Job drawing, mm, ordinate dimensions from the low corner. One solid piece. Give positions to 0.01 mm unless a question says otherwise; leave off trailing zeros. Order: outer loops, then holes, each group sorted by start corner. A loop starts at its lowest first (then second) coordinate and runs counter-clockwise, first axis right, second up. Notation, with made-up numbers: M 77,-21 L 119,-21 A17 cw 119,-8 Z; hole C 77.25,2 d2. An arc over 180 degrees is marked long. Put each result on its own line as item: value. Start each with the question number.
1) Cut at C-C (y = 16). Write the cut outline in (x, z) (1 decimal).
2) Cut at A-A (x = 17.5). Write the cut outline in (y, z).
3) Two-plate mould, pull along X, no slides. Class the marked faces 1, 2 and 3: released by +X, released by -X, zero draft, split by the parting line, or undercut.
4) Pin check, flat tips, straight feed: pin 1 (1.5 mm diameter, centred on x = 5.5, z = 22.5, fed in from -Y); pin 2 (12 mm diameter, centred on x = 21.5, z = 53, fed in from -Y); pin 3 (12 mm diameter, centred on x = 6.5, z = 60.5, fed in from -Y); pin 4 (10 mm diameter, centred on y = 54.5, z = 7, fed in from -X). Stop position of each tip, or through.
5) Drill centre lines: line 1 (Y direction, x = 32.5, z = 52) (1 decimal); line 2 (Y direction, x = 7, z = 22); line 3 (Z direction, x = 7, y = 14.5). Where is each one in solid material? Low to high. Write a range as [from, to].
6) Cut at B-B (z = 45). Write the cut outline in (x, y) (1 decimal).
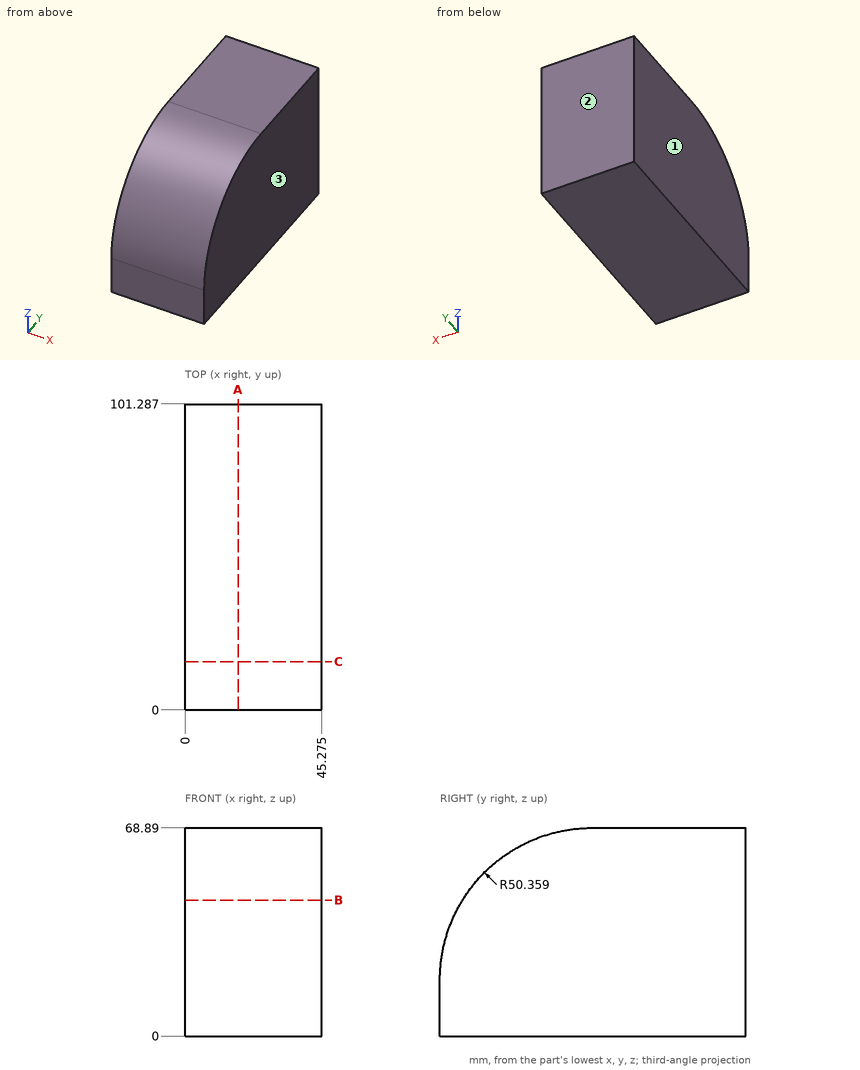
Solution:
1. outline: M 0,0 L 45.3,0 L 45.3,55.3 L 0,55.3 Z
2. outline: M 0,0 L 101.29,0 L 101.29,68.89 L 50.36,68.89 A50.36 ccw 0,18.53 Z
3. face 1: released by -X
3. face 2: zero draft
3. face 3: released by +X
4. pin 1: y = 0.1
4. pin 2: y = 8.82
4. pin 3: y = 15.11
4. pin 4: x = 0
5. line 1: [12.7, 101.3]
5. line 2: [0.12, 101.29]
5. line 3: [0, 53.89]
6. outline: M 0,7.5 L 45.3,7.5 L 45.3,101.3 L 0,101.3 Z
